Read the model definition and answer for the solid it produces. Units are mm, in the model's axes. A direction names the side the tool comes from. Round coordinates to 2 decimals unless told otherwise and drop trailing zeros. Write each loop counter-clockwise with the first axis right and the second up, starting at its lowest first coordinate (ties: lowest second). Pieces come first, ordered by that corner, then holes.
from build123d import *

# Parameters (mm, degrees)
F1_R      = 15.8036743057
F2_DEPTH  = 25.4
F0_W      = 31.5568223596
F0_H      = 33.1780388951
F3_DEPTH  = 25.4
F4_R      = 8.1334827116
F5_DEPTH  = 58.9108746499
F7_D      = 6.35
F9_D      = 25.4
F14_DEPTH = 25


# Not quite as in the source:
# - the program builds the solid bodies; features that only make, move or delete a surface that nothing else refers to are left out


with BuildPart() as f2:
    # F1 (on face) → F2 (new body)
    with BuildSketch(Plane.XY):
        with Locations((0, 33.3719775081)):
            Circle(F1_R)
    extrude(amount=F2_DEPTH)

    # F0 (on Top) → F3 (join)
    with BuildSketch(Plane.XY):
        with Locations((15.7784111798, 16.5890194476)):
            Rectangle(F0_W, F0_H)
    extrude(amount=F3_DEPTH)

    # F4 (on face) → F5 (join)
    with BuildSketch(Plane.XY.offset(25.4)):
        with Locations((0, 33.3719775081)):
            Circle(F4_R)
    extrude(amount=-F5_DEPTH)

    # F7 (through all)
    with Locations(Plane.XY.offset(25.4)):
        with Locations((0, 33.3719775081)):
            Hole(F7_D / 2)

    # F9 (through all)
    with Locations(Plane.XY.offset(25.4)):
        with Locations((17.5604298711, 14.967338182)):
            Hole(F9_D / 2)

    # F14 (add): a face of the model
    f14_faces = [f2.faces().sort_by_distance(p)[0] for p in [
        (15.7784111798, 0, 12.7),
    ]]
    extrude(f14_faces, amount=F14_DEPTH)


solid = f2.part
Q1. Section B-B (y = 31.5) is taken. Determine the outline of the cut face in (x, z).
Verdict:
outline: (-15.69, 0) - (-7.92, 0) - (-7.92, -33.51) - (-2.56, -33.51) - (-2.56, 25.4) - (-15.69, 25.4) - close; (2.56, -33.51) - (7.92, -33.51) - (7.92, 0) - (31.56, 0) - (31.56, 25.4) - (2.56, 25.4) - close
Q2. Determine the mould class of faces 1 (the cylindrical face through (-10.7, 45, 12.5)), 2 (the cylindrical face through (0.688, 30.272, -4.468)), 3 (the flat face through (31.557, 4, 13)), 4 (the flat face through (24, 33.178, 13)) for opening direction X: pulls with the +X half, pulls with the -X half, needs draft (parallel to the pull), parting line crosses it, or undercut.
Verdict:
face 1: parting line crosses it
face 2: undercut
face 3: pulls with the +X half
face 4: needs draft
Q3. Flat-ended cylindrical pins translate along their axes: pin 1 Ø1.5 at (x, z) = (10.5, -22) entering from -Y; pin 2 Ø6 at (y, z) = (20, 9.5) entering from -X; pin 3 Ø2 at (x, z) = (-0.5, -24.5) entering from -Y; pin 4 Ø23.5 at (x, y) = (17.5, 2.5) entering from -Z. Find the tip coordinate at first contact, or state that the pin passes through.
Verdict:
pin 1: passes through
pin 2: stops at x = -11.92
pin 3: stops at y = 25.24
pin 4: stops at z = 0
Q4. Straight lines are drawn through the part: probe 1 along Y at (x, z) = (0, -8); probe 2 along Y at (x, z) = (17.5, 21); probe 3 along Z at (x, y) = (-6, 20.5). For each, find the intervals that lie inside material, in ascending order.
Verdict:
probe 1: y = 25.24 to 30.2, 36.55 to 41.51
probe 2: y = -25 to 2.27, 27.67 to 33.18
probe 3: z = 0 to 25.4
Q5. Section D-D (x = -1.5) is taken. Determine the outline of the cut face in (y, z).
Verdict:
outline: (17.64, 0) - (25.38, 0) - (25.38, -33.51) - (30.57, -33.51) - (30.57, 25.4) - (17.64, 25.4) - close; (36.17, -33.51) - (41.37, -33.51) - (41.37, 0) - (49.1, 0) - (49.1, 25.4) - (36.17, 25.4) - close
Q6. Which of the six approach directions +Z, -Z, +X, -X, +Y, -Y give full straight-line access (tool end or side, diameter ignored) to faces 5 (the flat face through (4, 33, -33.511)), 6 (the cylindrical face through (-1.76, 25.43, -16.52)), 7 (the flat face through (0, -3, 13))?
Verdict:
face 5: -Z, +X, -X, +Y, -Y
face 6: -Z
face 7: +Z, -Z, -X, -Y
Q7. Section A-A (x = 28.5) is taken. Determine the outline of the cut face in (y, z).
Verdict:
outline: (-25, 0) - (8.52, 0) - (8.52, 25.4) - (-25, 25.4) - close; (21.42, 0) - (33.18, 0) - (33.18, 25.4) - (21.42, 25.4) - close
Q8. Section C-C (z = -3.5) is taken. Determine the outline of the cut face in (x, y) (3 decimals).
Verdict:
outline: circle Ø16.267 at (0, 33.372); hole circle Ø6.35 at (0, 33.372)
